Geometry: final body of the model. Coordinates: model frame, mm. A direction names the side the tool comes from. Round coordinates to 2 decimals unless told otherwise and drop trailing zeros. Loops run counter-clockwise (first coordinate to the right, second up) from the corner with the lowest first, then second, coordinate; pieces in that order, holes last. Notation, with made-up numbers: (65, 16.5) -> (79, 16.5) arc R30 cw to (79, 39.5) -> close; hole circle Ø5 at (-25, 15.5). An arc over 180 degrees is marked (long way). Answer in a Markdown table with one row per item.
Autodesk Inventor part; units mm, degrees
ref_plane "YZ Plane" through (0, 0, 0) normal (1, 0, 0) x (0, 1, 0)
ref_plane "XZ Plane" through (0, 0, 0) normal (0, 1, 0) x (-1, 0, 0)
ref_plane "XY Plane" through (0, 0, 0) normal (0, 0, 1) x (1, 0, 0)
sketch "Sketch1" plane through (0, 0, 0) normal (0, 0, 1) x (1, 0, 0)
  line L0 (-12.1708, 16.0073) -> (13.2292, 16.0073)
  line L1 (13.2292, 16.0073) -> (13.2292, -34.7927)
  line L2 (13.2292, -34.7927) -> (-12.1708, -34.7927)
  line L3 (-12.1708, -34.7927) -> (-12.1708, 16.0073)
  line L4 (11.9592, 14.7373) -> (-10.9008, 14.7373)
  line L5 (-10.9008, 14.7373) -> (-10.9008, -33.5227)
  line L6 (-10.9008, -33.5227) -> (11.9592, -33.5227)
  line L7 (11.9592, -33.5227) -> (11.9592, 14.7373)
  point P0 (0, 0)
  dimension "d0" = 25.4
  dimension "d1" = 50.8
  dimension "d2" = 1.27
extrude "Extrusion1" add sketch "Sketch1" along normal blind 190.5
sketch "Sketch2" plane through (-12.1708, 16.0073, 0) normal (0, 1, 0) x (1, 0, 0)
  circle A0 centre (12.7, -12.7) radius 1.7272
  line L0 (25.4, 0) -> (0, 0)
  line L1 (0, 0) -> (0, -190.5)
  point P0 (12.1708, 0)
  dimension "d5" = 3.4544
  dimension "d6" = 12.7
  dimension "d7" = 12.7
extrude "Extrusion2" cut sketch "Sketch2" against normal through all
pattern_linear "Rectangular Pattern1" count 19 spacing 25.4 along (0, 0, 1) of "Extrusion2"
sketch "Sketch5" plane through (-12.1708, -34.7927, 0) normal (-1, 0, 0) x (0, 0, 1)
  line L0 (0, 50.8) -> (0, 0)
  line L1 (139.7, 50.8) -> (190.5, 50.8)
  line L2 (190.5, 50.8) -> (190.5, 203.2)
  line L3 (190.5, 203.2) -> (139.7, 203.2)
  line L4 (139.7, 203.2) -> (139.7, 50.8)
  circle A0 centre (165.1, 101.6) radius 14.2875
  point P0 (0, 34.7927)
  point P1 (165.1, 50.8)
  dimension "d48" = 50.8
  dimension "d49" = 152.4
  dimension "d50" = 28.575
  dimension "d51" = 50.8
equation "\"d3\" = d13"
equation "\"d10\" = d14"
equation "\"d13\" = 190.5"
equation "\"d14\" = d13"
equation "\"d32\" = 101.6"
properties part number "ElevatorPivotBar2"
Item 1: Cut plane C-C (y = -29.5). Output: boundary loops of the cut face in (x, z), then the cut area to 3 significant figures.
Answer:
| item | result |
|---|---|
| outline | (-12.17, 0) -> (-10.9, 0) -> (-10.9, 190.5) -> (-12.17, 190.5) -> close; (11.96, 0) -> (13.23, 0) -> (13.23, 190.5) -> (11.96, 190.5) -> close |
| area | 484 mm² |
Item 2: Cut plane A-A (x = -8.5). Output: boundary loops of the cut face in (y, z), then the cut area to 3 significant figures.
Answer:
| item | result |
|---|---|
| outline | (-34.79, 0) -> (-33.52, 0) -> (-33.52, 190.5) -> (-34.79, 190.5) -> close; (14.74, 0) -> (16.01, 0) -> (16.01, 190.5) -> (14.74, 190.5) -> close |
| area | 484 mm² |
Item 3: Pin query (flat end, axial travel): pin 1 Ø3 at (x, z) = (0.53, 88.9) entering from -Y. Return the tip coordinate at first contact, or that it passes through.
Answer:
| item | result |
|---|---|
| pin 1 | passes through |
Item 4: Reachability of faces 1 (the face through (-10.901, -9, 94)), 2 (the face through (0.3, -34.15, 87.19)) from +Z, -Z, +X, -X, +Y, -Y: full face, straight path, thin tool, end or side. Return the list, or none.
Answer:
| item | result |
|---|---|
| face 1 | +Z, -Z |
| face 2 | +Y, -Y |
Item 5: Line query: probe 1 along Y at (x, z) = (10, 114.5); probe 2 along X at (y, z) = (-13, 52); probe 3 along X at (y, z) = (15.35, 12.7). Output: solid intervals per line, ascending. Write a range as [from, to].
Answer:
| item | result |
|---|---|
| probe 1 | y = [-34.79, -33.52], [14.74, 16.01] |
| probe 2 | x = [-12.17, -10.9], [11.96, 13.23] |
| probe 3 | x = [-12.17, -1.2], [2.26, 13.23] |
Item 6: Cut plane D-D (z = 100). Output: boundary loops of the cut face in (x, y), then the cut area to 3 significant figures.
Answer:
| item | result |
|---|---|
| outline | (-12.17, -34.79) -> (13.23, -34.79) -> (13.23, 16.01) -> (-12.17, 16.01) -> close; hole (-10.9, -33.52) -> (11.96, -33.52) -> (11.96, 14.74) -> (-10.9, 14.74) -> close |
| area | 187 mm² |
Item 7: Draft query along Z for faces 3 (the face through (0.3, 15.38, 87.19)), 4 (the face through (-12, -9, 0)), 5 (the face through (-11.2, -9.3, 190.5)). Return one class per face: pulls with the +Z half, pulls with the -Z half, needs draft (parallel to the pull), parting line crosses it, or undercut.
Answer:
| item | result |
|---|---|
| face 3 | undercut |
| face 4 | pulls with the -Z half |
| face 5 | pulls with the +Z half |
Item 8: Cut plane B-B (z = 139.7). Output: boundary loops of the cut face in (x, y), then the cut area to 3 significant figures.
Answer:
| item | result |
|---|---|
| outline | (-12.17, -34.79) -> (-1.2, -34.79) -> (-1.2, -33.52) -> (-10.9, -33.52) -> (-10.9, 14.74) -> (-1.2, 14.74) -> (-1.2, 16.01) -> (-12.17, 16.01) -> close; (2.26, -34.79) -> (13.23, -34.79) -> (13.23, 16.01) -> (2.26, 16.01) -> (2.26, 14.74) -> (11.96, 14.74) -> (11.96, -33.52) -> (2.26, -33.52) -> close |
| area | 178 mm² |
